Could you check a few things on this model? Use its own coordinates, in mm. A direction names the side the tool comes from. Give positions to 0.01 mm unless a question says otherwise; leave off trailing zeros. Order: outer loops, then holes, each group sorted by start corner. A loop starts at its lowest first (then second) coordinate and runs counter-clockwise, first axis right, second up. Notation, with made-up numbers: (0.5, 22.25) -> (21.5, 22.25) arc R15 ccw to (21.5, 48.25) -> close; hole circle Ø4 at (26.25, 8.25). An arc over 180 degrees is marked (long way). Use one line per item in the form item = value. Start each with the question number.
from build123d import *

# Parameters (mm, degrees)
EXTRUDE_1_DEPTH        = 10
EXTRUDE_2_DEPTH        = 2
EXTRUDE_2_DEPTH_BACK   = 2
SKETCH_4_W             = 1
SKETCH_4_H             = 10
CUT_EXTRUDE_2_DEPTH    = 1
PATTERN_LINEAR_2_COUNT = 10
PATTERN_LINEAR_2_PITCH = 2


with BuildPart() as part:
    # Эскиз1 → Бобышка-Вытянуть1 (new body)
    with BuildSketch(Plane(origin=(0, 0, 0), x_dir=(1, 0, 0), z_dir=(0, 1, 0))):
        Polygon((0, 0), (19.459034366, 20.826435939), (6.168868081, 20.826435939), (6.168868081, 63.073215602), (10.762186387, 63.073215602), (10.762186387, 67.42510234), (-10.697117185, 67.42510234), (-10.697117185, 63.073215602), (0, 63.073215602), align=None)
    extrude(amount=EXTRUDE_1_DEPTH)

    # Эскиз3 → Бобышка-Вытянуть2 (add, two sides: drawn at the far end of the back side and taken through both)
    with BuildSketch(Plane(origin=(0, 5, 0), x_dir=(-1, 0, 0), z_dir=(0, -1, 0)).offset(-EXTRUDE_2_DEPTH_BACK)):
        Polygon((9, 63.073215602), (0, 54.073215602), (0, 63.073215602), align=None)
    extrude(amount=EXTRUDE_2_DEPTH + EXTRUDE_2_DEPTH_BACK)

    # Эскиз4 → Вырез-Вытянуть2 (cut)
    with BuildSketch(Plane(origin=(0, 0, -67.42510234), x_dir=(-1, 0, 0), z_dir=(0, 0, -1))):
        with Locations((-9.262186387, 5)):
            Rectangle(SKETCH_4_W, SKETCH_4_H)
    cut_extrude_2 = extrude(amount=-CUT_EXTRUDE_2_DEPTH, mode=Mode.SUBTRACT)

    # Линейный массив2: Вырез-Вытянуть2 ×10
    with Locations(*[(-i * PATTERN_LINEAR_2_PITCH, 0, 0) for i in range(1, PATTERN_LINEAR_2_COUNT)]):
        add(cut_extrude_2, mode=Mode.SUBTRACT)


solid = part.part
(1) Which directions (+Z, -Z, +X, -X, +Y, -Y) give clear straight access to the entire face, cutting with the end or side of a thin tool? Please do faces 4 (the flat face through (-3, 7, -61)), 5 (the flat face through (-5.4, 2.7, -63.073)), 6 (the flat face through (-10, 5, -67.425)), 7 (the flat face through (-3, 3, -61)), 8 (the flat face through (8, 5, -63.073)).
(2) We'd pull the mould along Z, two halves only. Please class faces 1 (the flat face through (10.762, 5, -65)), 2 (the flat face through (-4.563, 5.028, -58.636)), 3 (the flat face through (13, 5, -20.826)): pulls with the +Z half, pulls with the -Z half, needs draft (parallel to the pull), parting line crosses it, or undercut.
(3) Imagine slicing it at B-B (x = 15). Write out the boundary of the cut face in (y, z).
(4) Imagine slicing it at A-A (z = -27). Write out the boundary of the cut face in (x, y).
(5) I'm going to push flat-ended pins straight in: pin 1 Ø6 at (x, z) = (7.5, -59.5) entering from -Y; pin 2 Ø4 at (x, y) = (-6.5, 7.5) entering from +Z; pin 3 Ø4 at (x, y) = (-2.5, 2) entering from +Z; pin 4 Ø0.5 at (y, z) = (5.5, -66.5) entering from +X. Where does each tip first touch, or does it pass through?
(6) Please list where these lines run through material, in increasing order: probe 1 along X at (y, z) = (9, -30); probe 2 along Z at (x, y) = (9, 9); probe 3 along Z at (x, y) = (-1.5, 9.5).
Calculated:
q1.face_4 = +Z, -X, +Y
q1.face_5 = +Z, -X
q1.face_6 = -Z, +X, -X, +Y, -Y
q1.face_7 = +Z, -X, -Y
q1.face_8 = +X, +Y, -Y
q2.face_1 = needs draft
q2.face_2 = pulls with the +Z half
q2.face_3 = undercut
q3.outline = (0, -20.83) -> (10, -20.83) -> (10, -16.05) -> (0, -16.05) -> close
q4.outline = (0, 0) -> (6.17, 0) -> (6.17, 10) -> (0, 10) -> close
q5.pin_1 = 0
q5.pin_2 = -58.64
q5.pin_3 = -54.84
q5.pin_4 = 10.76
q6.probe_1 = 0 to 6.17
q6.probe_2 = -66.43 to -63.07, -20.83 to -9.63
q6.probe_3 = -67.43 to -63.07
